from build123d import *

# Parameters (mm, degrees)
F0_R     = 50
F0_R_2   = 2.5
F0_R_3   = 15
F1_DEPTH = 20


with BuildPart() as f1:
    # F0 (on Top) → F1 (new body)
    with BuildSketch(Plane.XY):
        Circle(F0_R)
        with Locations((-29.698485, -29.698485)):
            Circle(F0_R_2, mode=Mode.SUBTRACT)
        with Locations((-18.384776, -18.384776)):
            Circle(F0_R_2, mode=Mode.SUBTRACT)
        with Locations((0, -42)):
            Circle(F0_R_2, mode=Mode.SUBTRACT)
        with Locations((0, -26)):
            Circle(F0_R_2, mode=Mode.SUBTRACT)
        with Locations((29.698485, -29.698485)):
            Circle(F0_R_2, mode=Mode.SUBTRACT)
        with Locations((18.384776, -18.384776)):
            Circle(F0_R_2, mode=Mode.SUBTRACT)
        with Locations((-42, 0)):
            Circle(F0_R_2, mode=Mode.SUBTRACT)
        with Locations((-26, 0)):
            Circle(F0_R_2, mode=Mode.SUBTRACT)
        with Locations((-18.384776, 18.384776)):
            Circle(F0_R_2, mode=Mode.SUBTRACT)
        with Locations((-29.698485, 29.698485)):
            Circle(F0_R_2, mode=Mode.SUBTRACT)
        Circle(F0_R_3, mode=Mode.SUBTRACT)
        with Locations((18.384776, 18.384776)):
            Circle(F0_R_2, mode=Mode.SUBTRACT)
        with Locations((26, 0)):
            Circle(F0_R_2, mode=Mode.SUBTRACT)
        with Locations((42, 0)):
            Circle(F0_R_2, mode=Mode.SUBTRACT)
        with Locations((0, 26)):
            Circle(F0_R_2, mode=Mode.SUBTRACT)
        with Locations((0, 42)):
            Circle(F0_R_2, mode=Mode.SUBTRACT)
        with Locations((29.698485, 29.698485)):
            Circle(F0_R_2, mode=Mode.SUBTRACT)
    extrude(amount=F1_DEPTH)


solid = f1.part
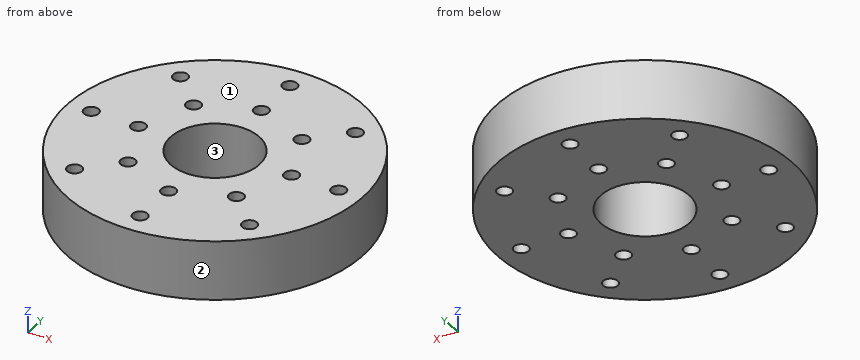
Could you check a few things on this model? Use its own coordinates, in mm. Face numbers are marked on the shaded views. Give positions to 0.01 mm unless a question says otherwise; leave off trailing zeros. Write each loop counter-clockwise with the first axis right and the second up, starting at its lowest first coordinate (ties: lowest second). Pieces come first, ordered by that corner, then holes. Notation, with made-up numbers: (1, 7.25) -> (52, 7.25) arc R10 ccw to (52, 11.25) -> close; hole circle Ø2 at (61, 43). An arc over 180 degrees is marked (long way). Answer as a JSON object with one key per item and string values.
Q1. Will these pins go through, and if not, where does the flat tip stop? pin 1 Ø8 at (x, z) = (0.5, 17.5) entering from +Y; pin 2 Ø10 at (x, z) = (-25.5, 2) entering from -Y; pin 3 Ø3 at (x, z) = (-36.5, 3.5) entering from +Y; pin 4 Ø6.5 at (x, y) = (29.7, -29.7) entering from -Z.
Taken from the geometry:
{"pin 1": "stops at y = 50", "pin 2": "stops at y = -45.6", "pin 3": "stops at y = 35.71", "pin 4": "stops at z = 0"}
Q2. We'd pull the mould along Y, two halves only. Please class the marked faces 1, 2 and 3: released by +Y, released by -Y, zero draft, split by the parting line, or undercut.
Taken from the geometry:
{"face 1": "zero draft", "face 2": "split by the parting line", "face 3": "undercut"}
Q3. Please list where these lines run through material, in increasing order: L1, parallel to Y at x = 0, z = 5; L2, parallel to Y at x = -17.5, z = 18.25; L3, parallel to Y at x = -20.5, z = 8.5.
Taken from the geometry:
{"L1": "y = -50 to -44.5, -39.5 to -28.5, -23.5 to -15, 15 to 23.5, 28.5 to 39.5, 44.5 to 50", "L2": "y = -46.84 to -20.72, -16.05 to 16.05, 20.72 to 46.84", "L3": "y = -45.6 to -19.72, -17.05 to 17.05, 19.72 to 45.6"}
Q4. Suppose I cut it at C-C on z = 3.25. Count the separate pieces of the cut face and the enclosed holes in it, then the cut area to 3 significant figures.
Taken from the geometry:
{"separate pieces": "1", "enclosed holes": "17", "area": "6,830 mm²"}
Q5. Suppose I cut it at A-A on x = -42. Write out the boundary of the cut face in (y, z).
Taken from the geometry:
{"outline": "(-27.13, 0) -> (-2.5, 0) -> (-2.5, 20) -> (-27.13, 20) -> close; (2.5, 0) -> (27.13, 0) -> (27.13, 20) -> (2.5, 20) -> close"}
